Work out the finished part from the listing and answer in its coordinate system (mm). A direction names the side the tool comes from. Give positions to 0.01 mm unless a question says otherwise; leave off trailing zeros. Loops run counter-clockwise (first coordinate to the right, second up) from the corner with the lowest first, then second, coordinate; pieces in that order, holes last. Notation, with made-up numbers: M -30.75,-17.75 L -12.75,-17.75 A22 ccw -12.75,21.25 Z; hole C -34,-11.5 d9. An arc over 180 degrees is marked long. Use a Markdown table: item, result.
```python
from build123d import *

# Parameters (mm, degrees)
SKETCH_R              = 26
SKETCH_R_2            = 6
PAD_DEPTH             = 1
SKETCH001_R           = 1.5
POCKET_DEPTH          = 148.092808
POLARPATTERN_COUNT    = 4
SKETCH002_R           = 1.5
POCKET001_DEPTH       = 148.092808
POLARPATTERN001_COUNT = 7
POLARPATTERN001_ANGLE = 270
POCKET002_DEPTH       = 1.001


with BuildPart() as part:
    # Sketch → Pad (new body)
    with BuildSketch(Plane.XY):
        Circle(SKETCH_R)
        Circle(SKETCH_R_2, mode=Mode.SUBTRACT)
    extrude(amount=PAD_DEPTH)

    # Sketch001 (on Face3 of Pad) → Pocket (cut, through all)
    with BuildSketch(Plane(origin=(0, 0, 0), x_dir=(1, 0, 0), z_dir=(0, 0, -1))):
        with Locations((0, 8)):
            Circle(SKETCH001_R)
    pocket = extrude(amount=-POCKET_DEPTH, mode=Mode.SUBTRACT)

    # PolarPattern: Pocket ×4 about axis
    polarpattern_axis = Axis((0, 0, 0), (0, 0, -1))
    for i in range(1, POLARPATTERN_COUNT):
        add(pocket.rotate(polarpattern_axis, i * 360 / POLARPATTERN_COUNT), mode=Mode.SUBTRACT)

    # Sketch002 (on Face2 of PolarPattern) → Pocket001 (cut, through all)
    with BuildSketch(Plane(origin=(0, 0, 0), x_dir=(1, 0, 0), z_dir=(0, 0, -1))):
        with Locations((0, 22)):
            Circle(SKETCH002_R)
    pocket001 = extrude(amount=-POCKET001_DEPTH, mode=Mode.SUBTRACT)

    # PolarPattern001: Pocket001 ×7 about axis
    polarpattern001_axis = Axis((0, 0, 0), (0, 0, -1))
    for i in range(1, POLARPATTERN001_COUNT):
        add(pocket001.rotate(polarpattern001_axis, i * POLARPATTERN001_ANGLE / (POLARPATTERN001_COUNT - 1)), mode=Mode.SUBTRACT)

    # Sketch003 (on Face2 of PolarPattern001) → Pocket002 (cut, through all)
    with BuildSketch(Plane(origin=(0, 0, 0), x_dir=(1, 0, 0), z_dir=(0, 0, -1))):
        with BuildLine():
            Line((10, 28.284271), (10, 14))
            ThreePointArc((10, 14), (10.215876, 12.703695), (10.840204, 11.54731))
            Line((10.840204, 11.54731), (-0.353553, 0.353553))
            Line((-0.353553, 0.353553), (0.353553, -0.353553))
            Line((0.353553, -0.353553), (11.54731, 10.840204))
            ThreePointArc((11.54731, 10.840204), (12.703695, 10.215876), (14, 10))
            Line((14, 10), (28.284271, 10))
            ThreePointArc((28.284271, 10), (21.213203, 21.213203), (10, 28.284271))
        make_face()
    extrude(amount=-POCKET002_DEPTH, mode=Mode.SUBTRACT)


solid = part.part
```
(1) Consider probe 1 along X at (y, z) = (0, 0.4); probe 2 along Y at (x, z) = (-16, 0.75). Determine where each line is inside the solid, lowest interval first. Write a range as [from, to].
Entries:
| item | result |
|---|---|
| probe 1 | x = [-26, -23.5], [-20.5, -9.5], [-6.5, -6], [6, 6.5], [9.5, 20.5], [23.5, 26] |
| probe 2 | y = [-20.49, -16.99], [-14.12, 14.12], [16.99, 20.49] |
(2) Which of the six approach directions +Z, -Z, +X, -X, +Y, -Y give full straight-line access (tool end or side, diameter ignored) to faces 1 (the flat face through (-0.36, 6.14, 0)), 2 (the flat face through (7.406, -8.113, 0.493))?
Entries:
| item | result |
|---|---|
| face 1 | -Z, +X, -X, +Y, -Y |
| face 2 | +Z, -Z |
(3) The mould has two halves that part along X. Classify faces 3 (the cylindrical face through (-17.66, 19.08, 0.49)), 4 (the flat face through (-0.36, 6.14, 1)), 5 (the cylindrical face through (-4.06, 4.42, 0.49)): released by +X, released by -X, zero draft, split by the parting line, or undercut.
Entries:
| item | result |
|---|---|
| face 3 | split by the parting line |
| face 4 | zero draft |
| face 5 | undercut |
(4) A cutting plane is placed at D-D (y = -22). Write down the section's boundary in (x, z), and give its area (3 significant figures).
Entries:
| item | result |
|---|---|
| outline | M -13.86,0 L -1.5,0 L -1.5,1 L -13.86,1 Z; M 1.5,0 L 10,0 L 10,1 L 1.5,1 Z |
| area | 20.9 mm² |
(5) A cutting plane is placed at C-C (y = -8). Write down the section's boundary in (x, z), and give its area (3 significant figures).
Entries:
| item | result |
|---|---|
| outline | M -24.74,0 L -1.5,0 L -1.5,1 L -24.74,1 Z; M 1.5,0 L 7.29,0 L 7.29,1 L 1.5,1 Z; M 8.71,0 L 24.74,0 L 24.74,1 L 8.71,1 Z |
| area | 45.1 mm² |
(6) A cutting plane is placed at A-A (y = 0). Write down the section's boundary in (x, z).
Entries:
| item | result |
|---|---|
| outline | M -26,0 L -23.5,0 L -23.5,1 L -26,1 Z; M -20.5,0 L -9.5,0 L -9.5,1 L -20.5,1 Z; M -6.5,0 L -6,0 L -6,1 L -6.5,1 Z; M 6,0 L 6.5,0 L 6.5,1 L 6,1 Z; M 9.5,0 L 20.5,0 L 20.5,1 L 9.5,1 Z; M 23.5,0 L 26,0 L 26,1 L 23.5,1 Z |
